Source: CAD feature listing. Evaluate the final solid. Frame: model axes, mm. A direction names the side the tool comes from. Coordinates: 2 decimals unless noted, no trailing zeros. Order: outer loops, then holes, each group sorted by start corner. A loop starts at its lowest first (then second) coordinate and runs counter-clockwise, first axis right, second up.
```python
from build123d import *

# Parameters (mm, degrees)
CROQUIS1_R                 = 7.95
SALIENTE_EXTRUIR1_DEPTH    = 7.5
CROQUIS2_R                 = 8.45
SALIENTE_EXTRUIR2_DEPTH    = 0.5
SALIENTE_EXTRUIR3_START    = -14.5
CROQUIS2_2_R               = 8.45
SALIENTE_EXTRUIR3_DEPTH    = 0.5
CROQUIS3_R                 = 5
SALIENTE_EXTRUIR4_DEPTH    = 21
CORTAR_EXTRUIR1_DEPTH      = 24.728779994
CORTAR_EXTRUIR1_DEPTH_BACK = 24.728779994
CROQUIS4_R                 = 3
CROQUIS7_W                 = 1.25
CROQUIS7_H                 = 5
CROQUIS9_W                 = 1.25
CROQUIS9_H                 = 8.45
CROQUIS10_R                = 4
CORTAR_EXTRUIR2_DEPTH      = 25.162057119


with BuildPart() as part:
    # Croquis1 → Saliente-Extruir1 (new, symmetric)
    with BuildSketch(Plane(origin=(0, 0, 0), x_dir=(-1, 0, 0), z_dir=(0, 1, 0))):
        with Locations(Location((0, 0, 0), (0, 0, 90))):
            Circle(CROQUIS1_R)
    extrude(amount=SALIENTE_EXTRUIR1_DEPTH, both=True)

    # Croquis2 → Saliente-Extruir2 (add)
    with BuildSketch(Plane(origin=(0, 7.5, 0), x_dir=(-1, 0, 0), z_dir=(0, 1, 0))):
        with Locations(Location((0, 0, 0), (0, 0, 90))):
            Circle(CROQUIS2_R)
    extrude(amount=-SALIENTE_EXTRUIR2_DEPTH)

    # Croquis2<2> → Saliente-Extruir3 (add)
    with BuildSketch(Plane(origin=(0, 7.5, 0), x_dir=(-1, 0, 0), z_dir=(0, 1, 0)).offset(SALIENTE_EXTRUIR3_START)):
        with Locations(Location((0, 0, 0), (0, 0, 90))):
            Circle(CROQUIS2_2_R)
    extrude(amount=-SALIENTE_EXTRUIR3_DEPTH)

    # Croquis3 → Saliente-Extruir4 (add)
    with BuildSketch(Plane(origin=(0, -7.5, 0), x_dir=(-1, 0, 0), z_dir=(0, 1, 0))):
        with Locations(Location((0, 0, 0), (0, 0, 270))):
            Circle(CROQUIS3_R)
    extrude(amount=SALIENTE_EXTRUIR4_DEPTH)

    # Croquis4 → Cortar-Extruir1 (cut, two sides: drawn at the far end of the back side and taken through both)
    with BuildSketch(Plane(origin=(0, -7, 0), x_dir=(-1, 0, 0), z_dir=(0, 1, 0)).offset(-CORTAR_EXTRUIR1_DEPTH_BACK)):
        with Locations(Location((0, 0, 0), (0, 0, 90))):
            Circle(CROQUIS4_R)
    extrude(amount=CORTAR_EXTRUIR1_DEPTH + CORTAR_EXTRUIR1_DEPTH_BACK, mode=Mode.SUBTRACT)

    # Croquis7 → Taladro roscado M32 (revolve, cut)
    with BuildSketch(Plane.ZX.offset(10.5)):
        with Locations((0.625, 2.5)):
            Rectangle(CROQUIS7_W, CROQUIS7_H)
    revolve(axis=Axis((-6.35, 10.5, 0), (1, 0, 0)), mode=Mode.SUBTRACT)

    # Croquis9 → Taladro roscado M31 (revolve, cut)
    with BuildSketch(Plane(origin=(0, 10.5, 0), x_dir=(0, 1, 0), z_dir=(1, 0, 0))):
        with Locations((0.625, 4.225)):
            Rectangle(CROQUIS9_W, CROQUIS9_H)
    revolve(axis=Axis((0, 10.5, -6.35), (0, 0, 1)), mode=Mode.SUBTRACT)

    # Croquis10 → Cortar-Extruir2 (cut, through all)
    with BuildSketch(Plane.XZ.offset(7.5)):
        with Locations(Location((0, 0, 0), (0, 0, 270))):
            Circle(CROQUIS10_R)
    extrude(amount=-CORTAR_EXTRUIR2_DEPTH, mode=Mode.SUBTRACT)


solid = part.part
```
1. Section query C-C, the plane y = 10.5. Output: boundary loops of the cut face in (x, z).
2. Access query for faces 1 (the cylindrical face through (4.406, 10.979, 1.155)), 2 (the cylindrical face through (2.54, -7.25, 8.06)), 3 (the flat face through (-3.1, 7, 7.5)), 4 (the cylindrical face through (-1.5, 10.46, -4.77)). Directions: +Z, -Z, +X, -X, +Y, -Y. A direction counts if a zero-diameter tool reaches every point of the face in a straight line with its end or side. Return the directions, or none.
3. Section query A-A, the plane z = 0. Output: boundary loops of the cut face in (x, y), plus the area to 3 significant figures.
4. Section query B-B, the plane x = 0. Output: boundary loops of the cut face in (y, z), plus the area to 3 significant figures.
5. Draft query along X for faces 5 (the flat face through (-4, 7.5, 4)), 6 (the cylindrical face through (-4.837, 0.098, -6.309)), 7 (the cylindrical face through (1.109, 11.077, 4.408)), 8 (the cylindrical face through (-3.549, 2.853, -1.846)). Return one class per face: +X half, -X half, draft (parallel to the pull), parting line (faces both ways), or undercut.
6. Contact query for flat-ended pins moving along their axis: P1, Ø9, axis at x = 0, z = 0, coming from the +Y side; P2, Ø4, axis at y = 10.5, z = 0, coming from the +X side; P3, Ø3, axis at x = -6, y = 0, coming from the +Z side; P4, Ø1.5, axis at y = 3, z = -4.5, coming from the +X side. Output: stop coordinate, or through.
7. Section query D-D, the plane x = 2. Output: boundary loops of the cut face in (y, z).
8. Material intervals for line 1 along Y through (x, z) = (4.35, 0); line 2 along Y through (x, z) = (-7.25, -3.5); line 3 along Y through (x, z) = (6.5, 3.5), sorted ascending.
Answer key:
1. outline: (-1.25, 3.8) - (-1.25, 4.84) arc R5 ccw (long way) to (4.84, -1.25) - (3.8, -1.25) arc R4 cw (long way) to start; (1.25, 3.8) arc R4 cw to (3.8, 1.25) - (4.84, 1.25) arc R5 ccw to (1.25, 4.84) - close
2. face 1: +X
2. face 2: +Y, -Y
2. face 3: none
2. face 4: +Y
3. outline: (-8.45, -7.5) - (-4, -7.5) - (-4, 13.5) - (-5, 13.5) - (-5, 7.5) - (-8.45, 7.5) - (-8.45, 7) - (-7.95, 7) - (-7.95, -7) - (-8.45, -7) - close; (4, -7.5) - (8.45, -7.5) - (8.45, -7) - (7.95, -7) - (7.95, 7) - (8.45, 7) - (8.45, 7.5) - (5, 7.5) - (5, 9.25) - (4, 9.25) - close; (4, 11.75) - (5, 11.75) - (5, 13.5) - (4, 13.5) - close
3. area: 129 mm2
4. outline: (-7.5, -8.45) - (-7, -8.45) - (-7, -7.95) - (7, -7.95) - (7, -8.45) - (7.5, -8.45) - (7.5, -5) - (13.5, -5) - (13.5, -4) - (-7.5, -4) - close; (-7.5, 4) - (9.25, 4) - (9.25, 5) - (7.5, 5) - (7.5, 8.45) - (7, 8.45) - (7, 7.95) - (-7, 7.95) - (-7, 8.45) - (-7.5, 8.45) - close; (11.75, 4) - (13.5, 4) - (13.5, 5) - (11.75, 5) - close
4. area: 129 mm2
5. face 5: draft
5. face 6: parting line
5. face 7: undercut
5. face 8: undercut
6. P1: stops at y = 13.5
6. P2: stops at x = 5
6. P3: stops at z = 6.55
6. P4: stops at x = 7.01
7. outline: (-7.5, -8.21) - (-7, -8.21) - (-7, -7.69) - (7, -7.69) - (7, -8.21) - (7.5, -8.21) - (7.5, -4.58) - (13.5, -4.58) - (13.5, -3.46) - (-7.5, -3.46) - close; (-7.5, 3.46) - (13.5, 3.46) - (13.5, 4.58) - (7.5, 4.58) - (7.5, 8.21) - (7, 8.21) - (7, 7.69) - (-7, 7.69) - (-7, 8.21) - (-7.5, 8.21) - close
8. line 1: y = -7.5 to 9.25, 11.75 to 13.5
8. line 2: y = -7.5 to -7, 7 to 7.5
8. line 3: y = -7.5 to 7.5
